from build123d import *

# Parameters (mm, degrees)
F0_R     = 17.65
F0_R_2   = 1.3
F0_W     = 9.2
F0_H     = 18.8
F1_DEPTH = 2


with BuildPart() as f1:
    # F0 (on Top) → F1 (new body)
    with BuildSketch(Plane.XY):
        Circle(F0_R)
        with Locations((0, -15.5)):
            Circle(F0_R_2, mode=Mode.SUBTRACT)
        with Locations((-15.5, 0)):
            Circle(F0_R_2, mode=Mode.SUBTRACT)
        Rectangle(F0_W, F0_H, mode=Mode.SUBTRACT)
        with Locations((15.5, 0)):
            Circle(F0_R_2, mode=Mode.SUBTRACT)
        with Locations((0, 15.5)):
            Circle(F0_R_2, mode=Mode.SUBTRACT)
    extrude(amount=F1_DEPTH)


solid = f1.part
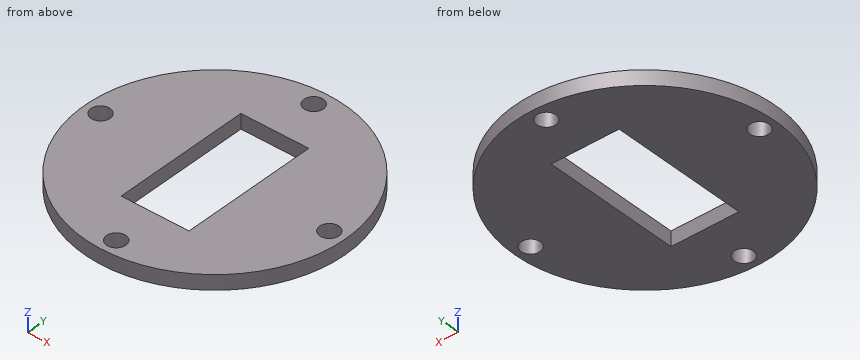
CAD build for the part. Positions are in the model's coordinates, mm. Give positions to 0.01 mm unless a question says otherwise; leave off trailing zeros. Loops run counter-clockwise (first coordinate to the right, second up) from the corner with the lowest first, then second, coordinate; pieces in that order, holes last. Notation, with made-up numbers: M 89,-19.75 L 111,-19.75 A28 ccw 111,1.25 Z; hole C 60.5,47 d4. An arc over 180 degrees is marked long. Answer in a Markdown table with one row per item. Add a question column.
Item 1: Drop flat-ended pins along their axis: P1, Ø2.5, axis at x = 15.5, y = 0, coming from the +Z side; P2, Ø0.6, axis at x = 1.5, z = 0.5, coming from the +Y side; P3, Ø1, axis at y = 4, z = 1.5, coming from the +X side; P4, Ø1, axis at x = -7, z = 1.5, coming from the -Y side. Give the stop position or say it passes through.
Item 2: Band-saw the part on B-B on x = 0. Give the cut face in (y, z), then the cut area to 3 significant figures.
Item 3: Band-saw the part on A-A on y = 0. Give the cut face in (x, z), then the cut area to 3 significant figures.
Item 4: Probe probe 1 along Y at (x, z) = (0, 0.6); probe 2 along X at (y, z) = (0.5, 0.3); probe 3 along X at (y, z) = (-1, 1.85). List the from-to ranges inside material, lowest first.
Item 5: Band-saw the part on D-D on x = 15.5. Give the cut face in (y, z).
Item 6: Band-saw the part on C-C on z = 0.55. Give the cut face in (x, y).
Reply:
| question | item | result |
|---|---|---|
| 1 | P1 | passes through |
| 1 | P2 | stops at y = 17.61 |
| 1 | P3 | stops at x = 17.3 |
| 1 | P4 | stops at y = -16.41 |
| 2 | outline | M -17.65,0 L -16.8,0 L -16.8,2 L -17.65,2 Z; M -14.2,0 L -9.4,0 L -9.4,2 L -14.2,2 Z; M 9.4,0 L 14.2,0 L 14.2,2 L 9.4,2 Z; M 16.8,0 L 17.65,0 L 17.65,2 L 16.8,2 Z |
| 2 | area | 22.6 mm^2 |
| 3 | outline | M -17.65,0 L -16.8,0 L -16.8,2 L -17.65,2 Z; M -14.2,0 L -4.6,0 L -4.6,2 L -14.2,2 Z; M 4.6,0 L 14.2,0 L 14.2,2 L 4.6,2 Z; M 16.8,0 L 17.65,0 L 17.65,2 L 16.8,2 Z |
| 3 | area | 41.8 mm^2 |
| 4 | probe 1 | y = -17.65 to -16.8, -14.2 to -9.4, 9.4 to 14.2, 16.8 to 17.65 |
| 4 | probe 2 | x = -17.64 to -16.7, -14.3 to -4.6, 4.6 to 14.3, 16.7 to 17.64 |
| 4 | probe 3 | x = -17.62 to -16.33, -14.67 to -4.6, 4.6 to 14.67, 16.33 to 17.62 |
| 5 | outline | M -8.44,0 L -1.3,0 L -1.3,2 L -8.44,2 Z; M 1.3,0 L 8.44,0 L 8.44,2 L 1.3,2 Z |
| 6 | outline | C 0,0 d35.3; hole C -15.5,0 d2.6; hole M -4.6,-9.4 L 4.6,-9.4 L 4.6,9.4 L -4.6,9.4 Z; hole C 0,-15.5 d2.6; hole C 0,15.5 d2.6; hole C 15.5,0 d2.6 |
